from build123d import *

# Parameters (mm, degrees)
F1_DEPTH    = 1.27
F2_R        = 0.0254
F4_DEPTH    = 0.508
F5_T1_DEPTH = 5.1142141328
F5_T3_DEPTH = 4.5716483018
F5_T5_DEPTH = 5.8519702279
F5_T7_DEPTH = 5.3913281872
F6_W        = 3.1516760678
F6_H        = 2.9446112536
F7_DEPTH    = 5.08
F8_T1_DEPTH = 7.62
F10_DEPTH   = 0.0254
F11_W       = 4.6949440148
F11_H       = 0.1139125334
F12_DEPTH   = 0.0254
F13_W       = 5.08
F13_H       = 0.9126112536
F14_DEPTH   = 0.508
F15_W       = 5.08
F15_H       = 0.9126112536
F16_DEPTH   = 0.508


# Not quite as in the source:
# - a fillet or chamfer that OpenCascade refuses, or shapes differently, is made with other operations: its cross-section is extruded or revolved along the edge and cut away or added


with BuildPart() as f1:
    # F0 (on Top) → F1 (new body, symmetric)
    with BuildSketch(Plane.XY):
        with BuildLine():
            Line((0.914706802, 2.159), (-1.879293198, 2.159))
            Line((-1.879293198, 2.159), (-1.879293198, -2.159))
            Line((-1.879293198, -2.159), (0.914706802, -2.159))
            Line((0.914706802, -2.159), (0.914706802, -0.889))
            Line((0.914706802, -0.889), (0.863906802, -0.889))
            Line((0.863906802, -0.889), (0.813106802, -0.889))
            ThreePointArc((0.813106802, -0.889), (-0.0443418563, -1.2221163224), (-0.901769336, -0.8889454908))
            ThreePointArc((-0.901769336, -0.8889454908), (-1.2648079256, 5.45092e-05), (-0.901769336, 0.8890545092))
            ThreePointArc((-0.901769336, 0.8890545092), (-0.0443206777, 1.2221708316), (0.813106802, 0.889))
            Line((0.813106802, 0.889), (0.863906802, 0.889))
            Line((0.863906802, 0.889), (0.914706802, 0.889))
            Line((0.914706802, 0.889), (0.914706802, 2.159))
        make_face()
    extrude(amount=F1_DEPTH, both=True)

    # F2
    f2_edges = [f1.edges().sort_by_distance(p)[0] for p in [
        (0.914707, 0.889, 0),
        (0.914707, -0.889, 0),
    ]]
    fillet(f2_edges, radius=F2_R)

    # F3 (on face) → F4 (join)
    with BuildSketch(Plane(origin=(-1.879293198, 0, 0), x_dir=(0, -1, 0), z_dir=(-1, 0, 0))):
        Polygon((-1.9648331217, 1.5023018932), (-2.159, 1.27), (-2.159, -1.27), (-1.9496894674, -1.5794709325), (1.8575610593, -1.5794709325), (2.159, -1.27), (2.159, 1.27), (1.8563199556, 1.5023018932), align=None)
    extrude(amount=F4_DEPTH)

    # F5: fillet of radius 2.794 on 4 edges, made by hand

    # F5_s2 → F5_t1 (cut)
    with BuildSketch(Plane.YZ.offset(-4.6904002644)):
        with BuildLine():
            ThreePointArc((1.0435902952, 1.5023018932), (1.6132619065, 1.4436099664), (2.159, 1.27))
            Line((2.159, 1.27), (1.9648331217, 1.5023018932))
            Line((1.9648331217, 1.5023018932), (1.0435902952, 1.5023018932))
        make_face()
    extrude(amount=F5_T1_DEPTH, mode=Mode.SUBTRACT)

    # F5_s4 → F5_t3 (cut)
    with BuildSketch(Plane.YZ.offset(-4.4191173489)):
        with BuildLine():
            ThreePointArc((-1.0435902952, 1.5023018932), (-1.6132619065, 1.4436099664), (-2.159, 1.27))
            Line((-2.159, 1.27), (-1.8563199556, 1.5023018932))
            Line((-1.8563199556, 1.5023018932), (-1.0435902952, 1.5023018932))
        make_face()
    extrude(amount=F5_T3_DEPTH, mode=Mode.SUBTRACT)

    # F5_s6 → F5_t5 (cut)
    with BuildSketch(Plane.YZ.offset(-5.0592783119)):
        with BuildLine():
            ThreePointArc((0.8808954219, -1.5794709325), (1.5384141613, -1.5010012872), (2.159, -1.27))
            Line((2.159, -1.27), (1.9496894674, -1.5794709325))
            Line((1.9496894674, -1.5794709325), (0.8808954219, -1.5794709325))
        make_face()
    extrude(amount=F5_T5_DEPTH, mode=Mode.SUBTRACT)

    # F5_s8 → F5_t7 (cut)
    with BuildSketch(Plane.YZ.offset(-4.8289572916)):
        with BuildLine():
            ThreePointArc((-2.159, -1.27), (-1.5384141613, -1.5010012872), (-0.8808954219, -1.5794709325))
            Line((-0.8808954219, -1.5794709325), (-1.8575610593, -1.5794709325))
            Line((-1.8575610593, -1.5794709325), (-2.159, -1.27))
        make_face()
    extrude(amount=F5_T7_DEPTH, mode=Mode.SUBTRACT)

    # F6 (on face) → F7 (join)
    with BuildSketch(Plane(origin=(-2.387293198, 0, 0), x_dir=(0, -1, 0), z_dir=(-1, 0, 0))):
        with Locations((-0.0374238726, -0.0286956604)):
            Rectangle(F6_W, F6_H)
    extrude(amount=F7_DEPTH)

    # F8: fillet of radius 1.016 on 4 edges, made by hand

    # F8_s2 → F8_t1 (cut)
    with BuildSketch(Plane.YZ.offset(-10.007293198)):
        with BuildLine():
            ThreePointArc((1.6132619065, 0.4276099664), (1.3156823962, 1.1460304561), (0.5972619065, 1.4436099664))
            Line((0.5972619065, 1.4436099664), (1.6132619065, 1.4436099664))
            Line((1.6132619065, 1.4436099664), (1.6132619065, 0.4276099664))
        make_face()
        with BuildLine():
            ThreePointArc((-1.5384141613, 0.4276099664), (-1.240834651, 1.1460304561), (-0.5224141613, 1.4436099664))
            Line((-0.5224141613, 1.4436099664), (-1.5384141613, 1.4436099664))
            Line((-1.5384141613, 1.4436099664), (-1.5384141613, 0.4276099664))
        make_face()
        with BuildLine():
            ThreePointArc((1.6132619065, -0.4850012872), (1.3156823962, -1.2034217769), (0.5972619065, -1.5010012872))
            Line((0.5972619065, -1.5010012872), (1.6132619065, -1.5010012872))
            Line((1.6132619065, -1.5010012872), (1.6132619065, -0.4850012872))
        make_face()
        with BuildLine():
            ThreePointArc((-1.5384141613, -0.4850012872), (-1.240834651, -1.2034217769), (-0.5224141613, -1.5010012872))
            Line((-0.5224141613, -1.5010012872), (-1.5384141613, -1.5010012872))
            Line((-1.5384141613, -1.5010012872), (-1.5384141613, -0.4850012872))
        make_face()
    extrude(amount=F8_T1_DEPTH, mode=Mode.SUBTRACT)

    # F9 (on face) → F10 (join)
    with BuildSketch(Plane.XY.offset(1.4436099664)):
        Polygon((-7.1662743576, 0.5972619065), (-7.1378163993, 0.466715981), (-2.5845263153, 0.466715981), (-2.609875286, 0.5972619065), align=None)
        Polygon((-2.5695776567, -0.5224141613), (-2.5845263153, -0.3768240858), (-7.1378163993, -0.3768240858), (-7.1378163993, -0.5224141613), align=None)
    extrude(amount=F10_DEPTH)

    # F11 (on face) → F12 (join)
    with BuildSketch(Plane(origin=(0, 0, -1.5010012872), x_dir=(1, 0, 0), z_dir=(0, 0, -1))):
        Polygon((-7.2172759101, 0.376087494), (-2.5223318953, 0.4174394126), (-2.5223318953, 0.5224141613), (-7.2172759101, 0.5224141613), align=None)
        with Locations((-4.8698039027, -0.5403056398)):
            Rectangle(F11_W, F11_H)
    extrude(amount=F12_DEPTH)

    # F13 (on face) → F14 (join)
    with BuildSketch(Plane(origin=(0, 1.6132619065, 0), x_dir=(-1, 0, 0), z_dir=(0, 1, 0))):
        with Locations((4.927293198, -0.0286956604)):
            Rectangle(F13_W, F13_H)
    extrude(amount=F14_DEPTH)

    # F15 (on face) → F16 (join)
    with BuildSketch(Plane.XZ.offset(1.5384141613)):
        with Locations((-4.927293198, -0.0286956604)):
            Rectangle(F15_W, F15_H)
    extrude(amount=F16_DEPTH)


solid = f1.part
Can you work these out from the model? Positions are in its coordinate system, mm. A direction names the side the tool comes from. Give positions to 0.01 mm unless a question says otherwise; leave off trailing zeros. Order: outer loops, then holes, each group sorted by start corner. A loop starts at its lowest first (then second) coordinate and runs counter-clockwise, first axis right, second up. Notation, with made-up numbers: M 16.25,28.5 L 69.25,28.5 A23 ccw 69.25,65.5 Z; hole C 9.25,26 d6. An arc over 180 degrees is marked long. One line per item, written item: value.
Item 1: If we section it at C-C on x = -6.5: Write out the boundary of the cut face in (y, z) (3 decimals), and give its area (3 significant figures).
Verdict:
outline: M -2.046,-0.485 L -1.538,-0.485 A1.016 ccw -0.522,-1.501 L -0.522,-1.526 L -0.382,-1.526 L -0.382,-1.501 L 0.483,-1.501 L 0.483,-1.526 L 0.597,-1.526 L 0.597,-1.501 A1.016 ccw 1.613,-0.485 L 2.121,-0.485 L 2.121,0.428 L 1.613,0.428 A1.016 ccw 0.597,1.444 L 0.597,1.469 L 0.467,1.469 L 0.467,1.444 L -0.377,1.444 L -0.377,1.469 L -0.522,1.469 L -0.522,1.444 A1.016 ccw -1.538,0.428 L -2.046,0.428 Z
area: 9.34 mm2
Item 2: If we mould it in two halves opening along Y, with no side actions, what happens to faces 1 (the face through (-1.265, -0.014, 0.018)), 2 (the face through (-1, 2.159, 0)), 3 (the face through (0.915, -2, 0)), 4 (the face through (-1, -2.159, 0))? For each: pulls with the +Y half, pulls with the -Y half, needs draft (parallel to the pull), parting line crosses it, or undercut.
Verdict:
face 1: undercut
face 2: pulls with the +Y half
face 3: needs draft
face 4: pulls with the -Y half
Item 3: Please list where these lines run through material, in increasing order: line 1 (Z direction, x = 0, y = -1.6); line 2 (Y direction, x = -5, z = -0.05); line 3 (X direction, y = -1.95, z = 0.6).
Verdict:
line 1: -1.27 to 1.27
line 2: -2.05 to 2.12
line 3: -2.39 to 0.91
Item 4: For faces 5 (the face through (-1.43, 0.03, -1.27)), 6 (the face through (-5, -2.046, 0)), 7 (the face through (-0.057, 1.222, 0.018)), 8 (the face through (-4.96, 1.32, -1.2)), which set-ups out of +Z, -Z, +X, -X, +Y, -Y let a thin tool reach every point of the face, with its end or its side?
Verdict:
face 5: -Z, +X, +Y, -Y
face 6: +Z, -Z, -X, -Y
face 7: +Z, -Z
face 8: -Z, -X, +Y
Item 5: If we section it at B-B on y = -0.2: Write out the boundary of the cut face in (x, z).
Verdict:
outline: M -7.47,-1.5 L -2.39,-1.5 L -2.39,-1.58 L -1.88,-1.58 L -1.88,-1.27 L -1.25,-1.27 L -1.25,1.27 L -1.88,1.27 L -1.88,1.5 L -2.39,1.5 L -2.39,1.44 L -7.47,1.44 Z
Item 6: For pin 1 (1.4 mm diameter, centred on x = -0.5, y = -0.5, fed in from +Z); pin 2 (1.5 mm diameter, centred on x = -4, y = -0.5, fed in from +Z), each with a flat end and sliding along its axis, tell me the tip position at first contact or that it passes through.
Verdict:
pin 1: z = 1.27
pin 2: z = 1.47
